Study the drawing (mm; zero at the part's minimum x, y, z) and answer. Round coordinates to 2 decimals unless told otherwise and drop trailing zeros. Loops run counter-clockwise (first coordinate to the right, second up) from the corner with the lowest first, then second, coordinate; pieces in that order, holes last. Notation, with made-up numbers: M 61,60.5 L 90,60.5 A19 ccw 90,92.5 Z; hole C 89.25,21 d1. An arc over 180 degrees is marked long. Put each result on its own line as item: value. Start each with the question number.
(1) Determine the mould class of the marked faces 1, 2 and 3 for opening direction Z: released by +Z, released by -Z, zero draft, split by the parting line, or undercut.
(2) Section A-A, the plane x = 4.5 is taken. Determine the outline of the cut face in (y, z).
(3) Section C-C, the plane y = 0.2 is taken. Determine the outline of the cut face in (x, z).
(4) A flat-ended cylindrical pin translates along its axis: P1, Ø1, axis at x = 5.5, z = 2.5, coming from the -Y side. Find the tip coordinate at first contact, or state that the pin passes through.
(5) Section B-B, the plane z = 4.5 is taken. Determine the outline of the cut face in (x, y).
(6) Straight lines are drawn through the part: line 1 (Z direction, x = 4.5, y = 0.4); line 2 (X direction, y = 0.15, z = 6.25); line 3 (X direction, y = 0.65, z = 5.5). For each, find the intervals that lie inside material, in ascending order.
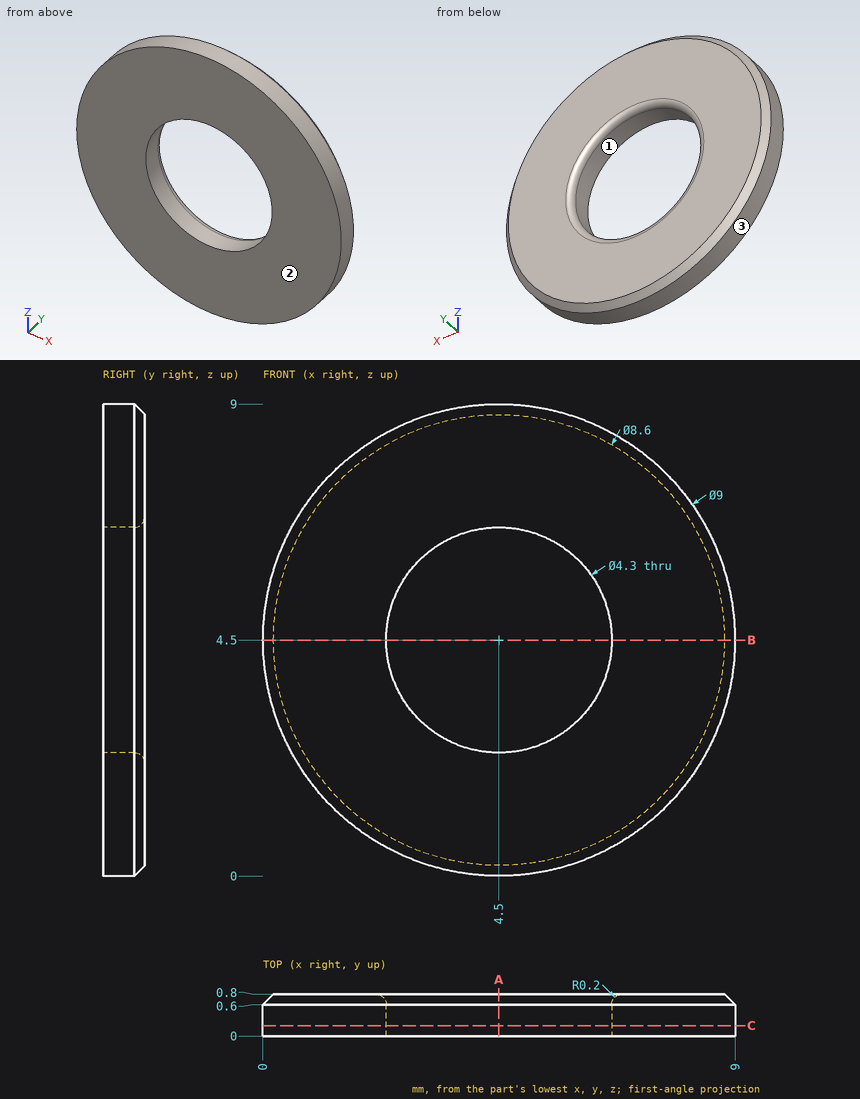
Recorded:
1. face 1: undercut
1. face 2: zero draft
1. face 3: split by the parting line
2. outline: M 0,0 L 0.6,0 L 0.8,0.2 L 0.8,2.15 A0.2 ccw 0.6,2.35 L 0,2.35 Z; M 0,6.65 L 0.6,6.65 A0.2 ccw 0.8,6.85 L 0.8,8.8 L 0.6,9 L 0,9 Z
3. outline: C 4.5,4.5 d9; hole C 4.5,4.5 d4.3
4. P1: stops at y = 0
5. outline: M 0,0 L 2.35,0 L 2.35,0.6 A0.2 ccw 2.15,0.8 L 0.2,0.8 L 0,0.6 Z; M 6.65,0 L 9,0 L 9,0.6 L 8.8,0.8 L 6.85,0.8 A0.2 ccw 6.65,0.6 Z
6. line 1: z = 0 to 2.35, 6.65 to 9
6. line 2: x = 0.35 to 3.25, 5.75 to 8.65
6. line 3: x = 0.16 to 2.59, 6.41 to 8.84
